Could you check a few things on this model? Use its own coordinates, in mm. A direction names the side the tool comes from. Round coordinates to 2 decimals unless told otherwise and drop trailing zeros. Loops run counter-clockwise (first coordinate to the right, second up) from the corner with the lowest first, then second, coordinate; pieces in that order, holes last. Notation, with made-up numbers: (22, -34) - (60, -34) arc R16 ccw to (60, -4) - close; hole circle Ø2 at (2.5, -26.75). An arc over 180 degrees is marked (long way). Use one line per item in the form item = value.
```python
from build123d import *

# Parameters (mm, degrees)
F0_R          = 7.5
F1_DEPTH      = 700
F2_R          = 5
F3_DEPTH      = 7.501
F3_DEPTH_BACK = 7.501
F5_R          = 17.5
F6_DEPTH      = 3
F7_R          = 17.5
F8_DEPTH      = 3


with BuildPart() as f1:
    # F0 (on Top) → F1 (new body)
    with BuildSketch(Plane.XY):
        Circle(F0_R)
    extrude(amount=F1_DEPTH)

    # F2 (on Right) → F3 (cut, two sides)
    with BuildSketch(Plane.YZ) as f3_sk:
        with Locations((0, 690)):
            Circle(F2_R)
    extrude(amount=-F3_DEPTH, mode=Mode.SUBTRACT)
    extrude(f3_sk.sketch, amount=F3_DEPTH_BACK, mode=Mode.SUBTRACT)

    # F5 (on Top) → F6 (join)
    with BuildSketch(Plane.XY):
        Circle(F5_R)
    extrude(amount=F6_DEPTH)

    # F7 (on offset) → F8 (join)
    with BuildSketch(Plane.XY.offset(100)):
        Circle(F7_R)
    extrude(amount=F8_DEPTH)


solid = f1.part
```
1. We'd pull the mould along Z, two halves only. Please class faces 1 (the face through (0, -8, 3)), 2 (the face through (0, 0, 700)), 3 (the face through (-13.887, -10.648, 101.479)), 4 (the face through (0, 0, 0)): +Z half, -Z half, draft (parallel to the pull), parting line (faces both ways), or undercut.
Solution:
face_1 = undercut
face_2 = +Z half
face_3 = draft
face_4 = -Z half
2. On a 3-axis mill with a long thin cutter (end or side, diameter ignored), from which of +Z, -Z, +X, -X, +Y, -Y can I reach the whole of each face in a straight line? I mean faces 5 (the face through (-7.493, 0.33, 397.321)), 6 (the face through (0, -8, 100)), 7 (the face through (-13.887, -10.648, 1.479)). Say none if no direction works.
Solution:
face_5 = +Z
face_6 = none
face_7 = +Z, -Z
3. For P1, Ø4, axis at y = 8.5, z = 236.5, coming from the +X side; P2, Ø10, axis at y = 13, z = 388, coming from the +X side; P3, Ø4, axis at x = -8.5, z = 465.5, coming from the +Y side; P4, Ø5, axis at x = 5, z = 210.5, coming from the -Y side, each with a flat end and sliding along its axis, tell me the tip position at first contact or that it passes through.
Solution:
P1 = 3.74
P2 = through
P3 = 3.74
P4 = -7.07
4. If we section it at A-A, the plane z = 63.5: Write out the boundary of the cut face in (x, y).
Solution:
outline = circle Ø15 at (0, 0)
5. Please list where these lines run through material, in increasing order: line 1 along Z through (x, y) = (3, 0); line 2 along Z through (x, y) = (-10, -11); line 3 along Y through (x, z) = (2.5, 690).
Solution:
line_1 = 0 to 685, 695 to 700
line_2 = 0 to 3, 100 to 103
line_3 = -7.07 to -5, 5 to 7.07
